from build123d import *

# Parameters (mm, degrees)
SKETCH1_R           = 23
BOSS_EXTRUDE1_DEPTH = 2
SKETCH3_R           = 0.5
CUT_EXTRUDE2_DEPTH  = 1
BOSS_EXTRUDE2_DEPTH = 5


with BuildPart() as part:
    # Sketch1 → Boss-Extrude1 (new body)
    with BuildSketch(Plane(origin=(0, 0, 0), x_dir=(1, 0, 0), z_dir=(0, 1, 0))):
        with Locations(Location((0, 0, 0), (0, 0, 270))):
            Circle(SKETCH1_R)
    extrude(amount=BOSS_EXTRUDE1_DEPTH)

    # Sketch3 → Cut-Extrude2 (cut)
    with BuildSketch(Plane(origin=(0, 0, 0), x_dir=(1, 0, 0), z_dir=(0, 1, 0))):
        with Locations(Location((0, 0, 0), (0, 0, 270))):
            Circle(SKETCH3_R)
    extrude(amount=CUT_EXTRUDE2_DEPTH, mode=Mode.SUBTRACT)

    # Sketch4 → Boss-Extrude2 (add)
    with BuildSketch(Plane(origin=(0, 0, 0), x_dir=(1, 0, 0), z_dir=(0, 1, 0))):
        with BuildLine():
            Line((0, 10.25), (0, 12.25))
            Line((0, 12.25), (-19.466317063, 12.25))
            ThreePointArc((-19.466317063, 12.25), (-23, 0), (-19.466317063, -12.25))
            Line((-19.466317063, -12.25), (0, -12.25))
            Line((0, -12.25), (0, -10.25))
            Line((0, -10.25), (-20.5, -10.25))
            Line((-20.5, -10.25), (-20.5, 10.25))
            Line((-20.5, 10.25), (0, 10.25))
        make_face()
    extrude(amount=BOSS_EXTRUDE2_DEPTH)


solid = part.part
Input: part model. Units: mm. Frame: model coordinates. A direction names the side the tool comes from. Round coordinates to 2 decimals unless told otherwise and drop trailing zeros. Order: outer loops, then holes, each group sorted by start corner. A loop starts at its lowest first (then second) coordinate and runs counter-clockwise, first axis right, second up. Notation, with made-up numbers: (-22.5, 2) - (7.5, 2) arc R20 cw to (7.5, 12) - close; hole circle Ø1 at (-23, 68.25). An arc over 180 degrees is marked (long way). Answer as a JSON object with one key per item and string values. Group by question number.
(1) Pin query (flat end, axial travel): P1, Ø0.8, axis at x = 0, z = 0, coming from the -Y side; P2, Ø1.5, axis at y = 4, z = -3.5, coming from the +X side; P3, Ø1, axis at y = 1.5, z = -4.5, coming from the +X side. Return the tip coordinate at first contact, or that it passes through.
(2) Cut plane C-C (x = -17.5). Return loops of the section in (y, z), then the cut area to 3 significant figures.
(3) Cut plane A-A (y = 3.8). Return loops of the section in (x, z).
(4) Draft query along X for faces 5 (the face through (-10, 3, 10.25)), 6 (the face through (-0.488, 0.493, -0.108)), 7 (the face through (-20.5, 3, 0)). Return one class per face: released by +X, released by -X, zero draft, split by the parting line, or undercut.
(5) Reachability of faces 1 (the face through (-10, 3, -12.25)), 2 (the face through (-10, 3, -10.25)), 3 (the face through (0, 3, -11)), 4 (the face through (-10, 3, 12.25)) from +Z, -Z, +X, -X, +Y, -Y: full face, straight path, thin tool, end or side. Return the list, or none.
(6) Cut plane B-B (z = 9). Return loops of the section in (x, y), then the cut area to 3 significant figures.
(7) Cut plane D-D (z = 2.5). Return loops of the section in (x, y).
(8) Material intervals for probe 1 along X at (y, z) = (0.4, 0); probe 2 along Z at (x, y) = (-8.5, 2.4), sorted ascending. Write a range as from..to.
Here are the results:
{
 "1": {"P1": "stops at y = 1", "P2": "stops at x = -20.5", "P3": "stops at x = 22.65"},
 "2": {"outline": "(0, -14.92) - (2, -14.92) - (2, -12.25) - (5, -12.25) - (5, -10.25) - (2, -10.25) - (2, 10.25) - (5, 10.25) - (5, 12.25) - (2, 12.25) - (2, 14.92) - (0, 14.92) - close", "area": "71.7 mm^2"},
 "3": {"outline": "(-20.5, -10.25) - (-20.5, 10.25) - (0, 10.25) - (0, 12.25) - (-19.47, 12.25) arc R23 ccw to (-19.47, -12.25) - (0, -12.25) - (0, -10.25) - close"},
 "4": {"face 5": "zero draft", "face 6": "undercut", "face 7": "released by +X"},
 "5": {"face 1": "-Z, +X, -X, +Y", "face 2": "+X, +Y", "face 3": "+Z, -Z, +X, +Y", "face 4": "+Z, +X, -X, +Y"},
 "6": {"outline": "(-21.17, 0) - (21.17, 0) - (21.17, 2) - (-20.5, 2) - (-20.5, 5) - (-21.17, 5) - close", "area": "86.7 mm^2"},
 "7": {"outline": "(-22.86, 0) - (22.86, 0) - (22.86, 2) - (-20.5, 2) - (-20.5, 5) - (-22.86, 5) - close"},
 "8": {"probe 1": "x = -23..-0.5, 0.5..23", "probe 2": "z = -12.25..-10.25, 10.25..12.25"}
}
